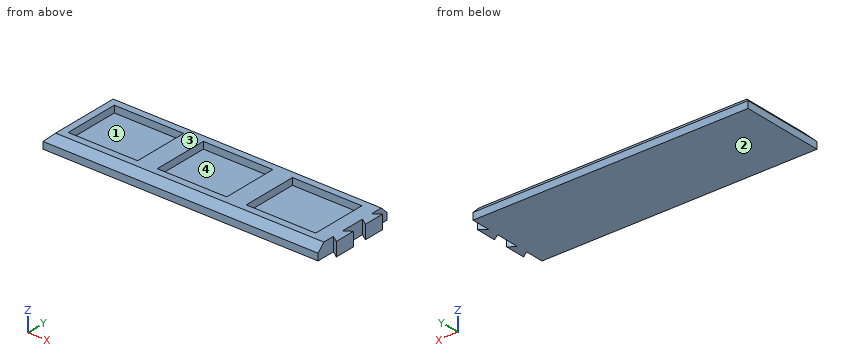
```python
from build123d import *

# Parameters (mm, degrees)
SKIZZE1_W                       = 200
SKIZZE1_H                       = 60.5
AUFSATZ_LINEAR_AUSTRAGEN1_DEPTH = 10
SKIZZE2_W                       = 50.5
SKIZZE2_H                       = 40.5
SCHNITT_LINEAR_AUSTRAGEN1_DEPTH = 5
FASE1_SIZE                      = 5
AUFSATZ_LINEAR_AUSTRAGEN2_DEPTH = 10


with BuildPart() as part:
    # Skizze1 → Aufsatz-Linear austragen1 (new body)
    with BuildSketch(Plane.XY):
        with Locations((100, 0)):
            Rectangle(SKIZZE1_W, SKIZZE1_H)
    extrude(amount=AUFSATZ_LINEAR_AUSTRAGEN1_DEPTH)

    # Skizze2 → Schnitt-Linear austragen1 (cut)
    with BuildSketch(Plane.XY.offset(10)):
        with Locations((35.25, 0)):
            Rectangle(SKIZZE2_W, SKIZZE2_H)
        with Locations((100, 0)):
            Rectangle(SKIZZE2_W, SKIZZE2_H)
        with Locations((164.75, 0)):
            Rectangle(SKIZZE2_W, SKIZZE2_H)
    extrude(amount=-SCHNITT_LINEAR_AUSTRAGEN1_DEPTH, mode=Mode.SUBTRACT)

    # Fase1
    fase1_edges = [part.edges().sort_by_distance(p)[0] for p in [
        (100, 30.25, 10),
        (0, 0, 10),
        (100, -30.25, 10),
    ]]
    chamfer(fase1_edges, length=FASE1_SIZE)

    # Skizze3 → Aufsatz-Linear austragen2 (add)
    with BuildSketch(Plane.XY.offset(10)):
        Polygon((200, 16.75), (205, 20.25), (205, 5.25), (200, 8.75), align=None)
        Polygon((200, -8.75), (205, -5.25), (205, -20.25), (200, -16.75), align=None)
    extrude(amount=-AUFSATZ_LINEAR_AUSTRAGEN2_DEPTH)


solid = part.part
```
Read the model definition and answer for the solid it produces. Units are mm, in the model's axes. Face numbers are marked on the shaded views. A direction names the side the tool comes from. Give positions to 0.01 mm unless a question says otherwise; leave off trailing zeros. Order: outer loops, then holes, each group sorted by start corner. A loop starts at its lowest first (then second) coordinate and runs counter-clockwise, first axis right, second up. Notation, with made-up numbers: (14.25, 85) -> (63.25, 85) arc R15 cw to (63.25, 98) -> close; hole circle Ø2 at (-38.5, -23). An arc over 180 degrees is marked (long way). One line per item, written item: value. Start each with the question number.
(1) Straight lines are drawn through the part: L1, parallel to X at y = -22.5, z = 5; L2, parallel to Z at x = 186.5, y = -5.5; L3, parallel to X at y = 17, z = 7. For each, find the intervals that lie inside material, in ascending order.
(2) For a pull along X with two mould halves and no side action, classify the marked faces 1 and 2 as released by +X, released by -X, zero draft, split by the parting line, or undercut.
(3) A tool of negligible diameter and unlimited length cuts with its end or side. For the marked faces 3 and 4, from which of +Z, -Z, +X, -X, +Y, -Y can it reach the whole face along a straight path? Write none if from no direction.
(4) The part is cut by section C-C (y = 14). Determine the outline of the cut face in (x, z).
(5) The part is cut by section D-D (y = -2.5). Determine the outline of the cut face in (x, z), and give its area (3 significant figures).
(6) Flat-ended cylindrical pins translate along their axes: P1, Ø1.5, axis at y = -7, z = 7.5, coming from the -X side; P2, Ø1.5, axis at y = 0.5, z = 8.5, coming from the -X side; P3, Ø5.5, axis at x = 110.5, z = 8, coming from the +Y side. Find the tip coordinate at first contact, or state that the pin passes through.
(7) The part is cut by section A-A (z = 7.5). Determine the outline of the cut face in (x, y).
(8) The part is cut by section B-B (x = 89). Determine the outline of the cut face in (y, z), and give its area (4 significant figures).
Taken from the geometry:
1. L1: 0 to 200
1. L2: 0 to 5
1. L3: 2 to 10, 60.5 to 74.75, 125.25 to 139.5, 190 to 200, 200.36 to 205
2. face 1: undercut
2. face 2: zero draft
3. face 3: +Z, +X, -X, +Y, -Y
3. face 4: +Z
4. outline: (0, 0) -> (205, 0) -> (205, 10) -> (190, 10) -> (190, 5) -> (139.5, 5) -> (139.5, 10) -> (125.25, 10) -> (125.25, 5) -> (74.75, 5) -> (74.75, 10) -> (60.5, 10) -> (60.5, 5) -> (10, 5) -> (10, 10) -> (5, 10) -> (0, 5) -> close
5. outline: (0, 0) -> (200, 0) -> (200, 10) -> (190, 10) -> (190, 5) -> (139.5, 5) -> (139.5, 10) -> (125.25, 10) -> (125.25, 5) -> (74.75, 5) -> (74.75, 10) -> (60.5, 10) -> (60.5, 5) -> (10, 5) -> (10, 10) -> (5, 10) -> (0, 5) -> close
5. area: 1,230 mm^2
6. P1: x = 1.75
6. P2: x = 2.75
6. P3: y = 30
7. outline: (2.5, -27.75) -> (200, -27.75) -> (200, -16.75) -> (205, -20.25) -> (205, -5.25) -> (200, -8.75) -> (200, 8.75) -> (205, 5.25) -> (205, 20.25) -> (200, 16.75) -> (200, 27.75) -> (2.5, 27.75) -> close; hole (10, -20.25) -> (60.5, -20.25) -> (60.5, 20.25) -> (10, 20.25) -> close; hole (74.75, -20.25) -> (125.25, -20.25) -> (125.25, 20.25) -> (74.75, 20.25) -> close; hole (139.5, -20.25) -> (190, -20.25) -> (190, 20.25) -> (139.5, 20.25) -> close
8. outline: (-30.25, 0) -> (30.25, 0) -> (30.25, 5) -> (25.25, 10) -> (20.25, 10) -> (20.25, 5) -> (-20.25, 5) -> (-20.25, 10) -> (-25.25, 10) -> (-30.25, 5) -> close
8. area: 377.5 mm^2
